Source: CAD feature listing. Evaluate the final solid. Frame: model axes, mm. A direction names the side the tool comes from. Give positions to 0.01 mm unless a question says otherwise; leave off trailing zeros. Loops run counter-clockwise (first coordinate to the right, second up) from the corner with the lowest first, then second, coordinate; pieces in that order, holes last. Notation, with made-up numbers: (6.25, -9) - (53.25, -9) arc R21 ccw to (53.25, 21) - close; hole circle Ø2 at (62, 37). An arc over 180 degrees is marked (long way). Put each result on its own line as item: value.
Autodesk Inventor part; units mm, degrees
ref_plane "YZ Plane" through (0, 0, 0) normal (1, 0, 0) x (0, 1, 0)
ref_plane "XZ Plane" through (0, 0, 0) normal (0, 1, 0) x (-1, 0, 0)
ref_plane "XY Plane" through (0, 0, 0) normal (0, 0, 1) x (1, 0, 0)
sketch "Szkic1" plane through (0, 0, 0) normal (0, 1, 0) x (-1, 0, 0)
  line L0 (-50, -50) -> (50, -50)
  line L1 (50, -50) -> (50, 50)
  line L2 (50, 50) -> (-50, 50)
  line L3 (-50, 50) -> (-50, -50)
  line L4 (-50, -50) -> (50, 50) construction
  line L5 (50, -50) -> (-50, 50) construction
  point P0 (0, 0)
  dimension "d0" = 100
  dimension "d1" = 100
extrude "Wyciągnięcie proste1" add sketch "Szkic1" along normal blind 100
sketch "Szkic2" plane through (0, 100, 0) normal (0, 1, 0) x (1, 0, 0)
  line L0 (46, -46) -> (-46, -46)
  line L1 (-46, -46) -> (-46, 46)
  line L2 (-46, 46) -> (46, 46)
  line L3 (46, 46) -> (46, -46)
  line L4 (46, -46) -> (-46, 46) construction
  line L5 (-46, -46) -> (46, 46) construction
  point P0 (0, 0)
  dimension "d4" = 92
  dimension "d5" = 92
extrude "Wyciągnięcie proste2" cut sketch "Szkic2" against normal blind 100
sketch "Szkic3" plane through (0, 0, 0) normal (0, -1, 0) x (1, 0, 0)
  line L0 (-48, -48) -> (48, -48)
  line L1 (48, -48) -> (48, 48)
  line L2 (48, 48) -> (-48, 48)
  line L3 (-48, 48) -> (-48, -48)
  line L4 (-48, -48) -> (48, 48) construction
  line L5 (48, -48) -> (-48, 48) construction
  line L6 (-46, -46) -> (46, -46)
  line L7 (46, -46) -> (46, 46)
  line L8 (46, 46) -> (-46, 46)
  line L9 (-46, 46) -> (-46, -46)
  line L10 (-46, -46) -> (46, 46) construction
  line L11 (46, -46) -> (-46, 46) construction
  point P0 (0, 0)
  dimension "d8" = 96
  dimension "d9" = 96
  dimension "d10" = 92
  dimension "d11" = 92
extrude "Wyciągnięcie proste3" add sketch "Szkic3" along normal blind 10 contours L3 L2 L1 L0 | L9 L8 L7 L6
sketch "Szkic4" plane through (0, -10, 0) normal (0, -1, 0) x (1, 0, 0)
  line L0 (46, 46) -> (-46, 46)
  line L1 (-46, 46) -> (-46, -46)
  line L2 (-46, -46) -> (46, -46)
  line L3 (46, -46) -> (46, 46)
  line L4 (46, 46) -> (-46, -46) construction
  line L5 (-46, 46) -> (46, -46) construction
  point P0 (0, 0)
  dimension "d14" = 92
  dimension "d15" = 92
extrude "Wyciągnięcie proste4" cut sketch "Szkic4" against normal blind 10
sketch "Szkic5" plane through (0, 100, 0) normal (0, 1, 0) x (1, 0, 0)
  line L0 (-2, 46) -> (2, 46)
  line L1 (2, 46) -> (2, -46)
  line L2 (2, -46) -> (-2, -46)
  line L3 (-2, -46) -> (-2, 46)
  line L4 (-2, 46) -> (2, -46) construction
  line L5 (2, 46) -> (-2, -46) construction
  point P0 (0, 0)
  dimension "d18" = 4
  dimension "d19" = 92
extrude "Wyciągnięcie proste5" add sketch "Szkic5" against normal blind 10
sketch "Szkic6" plane through (0, 100, 0) normal (0, 1, 0) x (1, 0, 0)
  line L0 (46, 46) -> (46, -46)
  line L1 (2, 46) -> (46, 46)
  line L2 (50, 50) -> (-50, 50)
  line L3 (50, -50) -> (50, 50)
  line L4 (2, -46) -> (2, 46)
  point P0 (0, 0)
  point P1 (46, 0)
fillet "Zaokrąglenie1" radius 4 16 edges at (2, 95, 46) (2, 95, -46) (-2, 95, -46) (-2, 95, 46) (50, 50, 50) (-50, 50, 50) (-50, 50, -50) (50, 50, -50) (46, 45, -46) (46, 45, 46) (-46, 45, 46) (-46, 45, -46) (-48, -5, 48) (48, -5, 48) (48, -5, -48) (-48, -5, -48)
equation "\"PromieńGięcia\" = Grubość"
equation "\"SzerokośćGięciaPodcięcia\" = Grubość"
equation "\"GłębokośćGięciaPodcięcia\" = 0.5 * Grubość"
equation "\"RozmiarPodcięciaNarożnika\" = 4 * Grubość"
equation "\"MinimalnaPozostałość\" = 2 * Grubość"
equation "\"PromieńPrzejścia\" = PromieńGięcia"
equation "\"Rozmiar_promienia_Jacobiego\" = PromieńGięcia"
equation "\"Wielk_odstępu\" = Grubość"
1) Access query for faces 1 (the cylindrical face through (-44.859, 44.23, -44.797)), 2 (the cylindrical face through (-46.859, -5.07, -46.797)), 3 (the flat face through (-1, -5, -48)), 4 (the cylindrical face through (-48.859, 50.7, 48.797)), 5 (the cylindrical face through (-46.797, -5.07, 46.859)). Directions: +Z, -Z, +X, -X, +Y, -Y. A direction counts if a zero-diameter tool reaches every point of the face in a straight line with its end or side. Return the directions, or none.
Check result:
face 1: +Y, -Y
face 2: -Z, -X, -Y
face 3: -Z, +X, -X, -Y
face 4: +Z, -X, +Y, -Y
face 5: +Z, -X, -Y
2) Section query A-A, the plane y = 84. Output: boundary loops of the cut face in (x, z), plus the area to 3 significant figures.
Check result:
outline: (-50, -46) arc R4 ccw to (-46, -50) - (46, -50) arc R4 ccw to (50, -46) - (50, 46) arc R4 ccw to (46, 50) - (-46, 50) arc R4 ccw to (-50, 46) - close; hole (-46, -42) arc R4 ccw to (-42, -46) - (42, -46) arc R4 ccw to (46, -42) - (46, 42) arc R4 ccw to (42, 46) - (-42, 46) arc R4 ccw to (-46, 42) - close
area: 1,540 mm²
3) Pin query (flat end, axial travel): P1, Ø11, axis at x = 8, y = -7, coming from the -Z side; P2, Ø3, axis at y = -7.5, z = -3, coming from the +X side; P3, Ø8, axis at x = -21, y = -4.5, coming from the +Z side. Return the tip coordinate at first contact, or that it passes through.
Check result:
P1: z = -48
P2: x = 48
P3: z = 48
4) Section query C-C, the plane x = 7.5. Output: boundary loops of the cut face in (y, z).
Check result:
outline: (-10, -48) - (0, -48) - (0, -50) - (100, -50) - (100, -46) - (-10, -46) - close; (-10, 46) - (100, 46) - (100, 50) - (0, 50) - (0, 48) - (-10, 48) - close
5) Material intervals for line 1 along X through (y, z) = (92, -22.5); line 2 along Z through (x, y) = (32.5, 44.5), sorted ascending. Write a range as [from, to].
Check result:
line 1: [-50, -46], [-2, 2], [46, 50]
line 2: [-50, -46], [46, 50]
6) Section query B-B, the plane z = -22.5. Output: boundary loops of the cut face in (x, y).
Check result:
outline: (-50, 0) - (-48, 0) - (-48, -10) - (-46, -10) - (-46, 100) - (-50, 100) - close; (-2, 90) - (2, 90) - (2, 100) - (-2, 100) - close; (46, -10) - (48, -10) - (48, 0) - (50, 0) - (50, 100) - (46, 100) - close
7) Mould query, pull axis X, two halves, no side actions, for faces 6 (the cylindrical face through (3.203, 94.93, 44.859)), 7 (the flat face through (48, -5, -1)), 8 (the flat face through (48.4, 0, 22.5)). Classes: pulls with the +X half, pulls with the -X half, needs draft (parallel to the pull), parting line crosses it, or undercut.
Check result:
face 6: undercut
face 7: pulls with the +X half
face 8: needs draft
